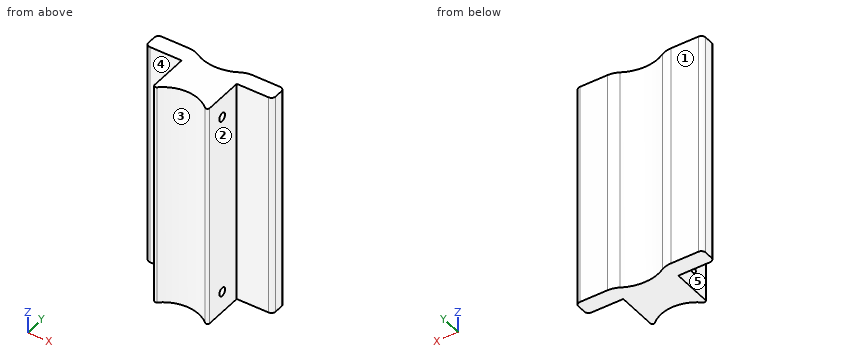
from build123d import *

# Parameters (mm, degrees)
AUFSATZ_LINEAR_AUSTRAGEN1_DEPTH = 106.5
SKIZZE2_R                       = 20
SCHNITT_LINEAR_AUSTRAGEN1_DEPTH = 118.653091757
VERRUNDUNG1_R                   = 10
VERRUNDUNG2_R                   = 2
VERRUNDUNG3_R                   = 1
SKIZZE3_R                       = 2
SCHNITT_LINEAR_AUSTRAGEN2_DEPTH = 122.619283011


with BuildPart() as part:
    # Skizze1 → Aufsatz-Linear austragen1 (new body)
    with BuildSketch(Plane.XY):
        with BuildLine():
            Line((-30, 32), (-13, 32))
            Line((-13, 32), (-13, 10.95445115))
            ThreePointArc((-13, 10.95445115), (0, 17), (13, 10.95445115))
            Line((13, 10.95445115), (13, 32))
            Line((13, 32), (30, 32))
            Line((30, 32), (30, 40))
            Line((30, 40), (-30, 40))
            Line((-30, 40), (-30, 32))
        make_face()
    extrude(amount=AUFSATZ_LINEAR_AUSTRAGEN1_DEPTH)

    # Skizze2 → Schnitt-Linear austragen1 (cut, through all)
    with BuildSketch(Plane(origin=(0, 0, 0), x_dir=(-1, 0, 0), z_dir=(0, 0, -1))):
        with Locations((0, 56)):
            Circle(SKIZZE2_R)
    extrude(amount=-SCHNITT_LINEAR_AUSTRAGEN1_DEPTH, mode=Mode.SUBTRACT)

    # Verrundung1
    verrundung1_edges = [part.edges().sort_by_distance(p)[0] for p in [
        (-12, 40, 53.25),
        (12, 40, 53.25),
    ]]
    fillet(verrundung1_edges, radius=VERRUNDUNG1_R)

    # Verrundung2
    verrundung2_edges = [part.edges().sort_by_distance(p)[0] for p in [
        (-30, 40, 53.25),
        (30, 40, 53.25),
        (30, 32, 53.25),
        (-30, 32, 53.25),
    ]]
    fillet(verrundung2_edges, radius=VERRUNDUNG2_R)

    # Verrundung3
    verrundung3_edges = [part.edges().sort_by_distance(p)[0] for p in [
        (13, 10.95445115, 53.25),
        (-13, 10.95445115, 53.25),
    ]]
    fillet(verrundung3_edges, radius=VERRUNDUNG3_R)

    # Skizze3 → Schnitt-Linear austragen2 (cut, through all)
    with BuildSketch(Plane(origin=(13, 0, 0), x_dir=(0, 0, -1), z_dir=(1, 0, 0))):
        with Locations(Location((-10, 22, 0), (0, 0, 90))):
            Circle(SKIZZE3_R)
        with Locations(Location((-96.5, 22, 0), (0, 0, 90))):
            Circle(SKIZZE3_R)
    extrude(amount=-SCHNITT_LINEAR_AUSTRAGEN2_DEPTH, mode=Mode.SUBTRACT)


solid = part.part
Verification items for the finished model (mm, model axes). Face numbers are marked on the shaded views. A direction names the side the tool comes from. Give positions to 0.01 mm unless a question says otherwise; leave off trailing zeros. Loops run counter-clockwise (first coordinate to the right, second up) from the corner with the lowest first, then second, coordinate; pieces in that order, holes last. Notation, with made-up numbers: (52.5, 89.25) - (59.5, 89.25) arc R26 ccw to (59.5, 112.25) - close; hole circle Ø10 at (18, 44). An arc over 180 degrees is marked (long way). Write each question's results on one line, items separated by ' | '.
1) Sectioned sample at B-B on y = 22. Record the boundary of the cut face in (x, z).
Solution:
outline: (-13, 0) - (13, 0) - (13, 8) - (-13, 8) - close; (-13, 12) - (13, 12) - (13, 94.5) - (-13, 94.5) - close; (-13, 98.5) - (13, 98.5) - (13, 106.5) - (-13, 106.5) - close
2) Material ranges on L1, parallel to Z at x = -4.75, y = 22; L2, parallel to Z at x = -2.5, y = 20.25; L3, parallel to X at y = 13.75, z = 44, recorded low to high. Write a range as from..to.
Solution:
L1: 0..8, 12..94.5, 98.5..106.5 | L2: 0..9.03, 10.97..95.53, 97.47..106.5 | L3: -13..-10, 10..13
3) Depth check by flat-ended pin: P1, Ø1, axis at x = -8, z = 43.5, coming from the +Y side; P2, Ø6, axis at x = -20, z = 40.5, coming from the -Y side; P3, Ø5, axis at y = 22, z = 96.5, coming from the -X side. Enter the tip coordinate at first touch or a pass-through.
Solution:
P1: y = 37.9 | P2: y = 32 | P3: x = -13
4) Mould release check, pull along X, two halves, no side actions. Record for the marked faces 3, 4 and 5: pulls with the +X half, pulls with the -X half, needs draft (parallel to the pull), parting line crosses it, or undercut.
Solution:
face 3: undercut | face 4: needs draft | face 5: pulls with the -X half
5) Sectioned sample at C-C on z = 29.5. Record the boundary of the cut face in (x, y).
Solution:
outline: (-30, 34) arc R2 ccw to (-28, 32) - (-13, 32) - (-13, 13.42) arc R1 ccw to (-11.33, 12.67) arc R17 cw to (11.33, 12.67) arc R1 ccw to (13, 13.42) - (13, 32) - (28, 32) arc R2 ccw to (30, 34) - (30, 38) arc R2 ccw to (28, 40) - (14.97, 40) arc R10 ccw to (9.98, 38.67) arc R20 cw to (-9.98, 38.67) arc R10 ccw to (-14.97, 40) - (-28, 40) arc R2 ccw to (-30, 38) - close
6) Tool access check on the marked faces 1 and 2. Record the directions out of +Z, -Z, +X, -X, +Y, -Y that give a thin tool (end or side, any length) a straight path to the whole face; none if there is none.
Solution:
face 1: +Z, -Z, +X, -X, +Y | face 2: +Z, -Z, +X, -Y
7) Sectioned sample at A-A on z = 10. Record the boundary of the cut face in (x, y).
Solution:
outline: (-30, 34) arc R2 ccw to (-28, 32) - (-13, 32) - (-13, 24) - (13, 24) - (13, 32) - (28, 32) arc R2 ccw to (30, 34) - (30, 38) arc R2 ccw to (28, 40) - (14.97, 40) arc R10 ccw to (9.98, 38.67) arc R20 cw to (-9.98, 38.67) arc R10 ccw to (-14.97, 40) - (-28, 40) arc R2 ccw to (-30, 38) - close; (-13, 13.42) arc R1 ccw to (-11.33, 12.67) arc R17 cw to (11.33, 12.67) arc R1 ccw to (13, 13.42) - (13, 20) - (-13, 20) - close
8) Sectioned sample at D-D on x = 0.5. Record the boundary of the cut face in (y, z).
Solution:
outline: (16.99, 0) - (36.01, 0) - (36.01, 106.5) - (16.99, 106.5) - close; hole circle Ø4 at (22, 10); hole circle Ø4 at (22, 96.5)
